```python
from build123d import *

# Parameters (mm, degrees)
SKETCH1_W           = 30
SKETCH1_H           = 99.95
BOSS_EXTRUDE1_DEPTH = 3.75
SKETCH2_W           = 30
SKETCH2_H           = 5
BOSS_EXTRUDE2_DEPTH = 20
SKETCH3_W           = 30
SKETCH3_H           = 5
BOSS_EXTRUDE3_DEPTH = 10
FILLET1_R           = 10
FILLET2_R           = 10


with BuildPart() as part:
    # Sketch1 → Boss-Extrude1 (new, symmetric)
    with BuildSketch(Plane.XY):
        with Locations((0, 49.975)):
            Rectangle(SKETCH1_W, SKETCH1_H)
    extrude(amount=BOSS_EXTRUDE1_DEPTH, both=True)

    # Sketch2 → Boss-Extrude2 (add, symmetric)
    with BuildSketch(Plane.XY):
        with Locations((0, 2.5)):
            Rectangle(SKETCH2_W, SKETCH2_H)
    extrude(amount=BOSS_EXTRUDE2_DEPTH, both=True)

    # Sketch3 → Boss-Extrude3 (add, symmetric)
    with BuildSketch(Plane.XY):
        with Locations((0, 97.45)):
            Rectangle(SKETCH3_W, SKETCH3_H)
    extrude(amount=BOSS_EXTRUDE3_DEPTH, both=True)

    # Fillet1
    # the kernel refuses this fillet: 10 mm, written as the material it adds along each edge
    with BuildSketch(Plane(origin=(15, 94.95, -3.75), x_dir=(0, 0, -1), z_dir=(-1, 0, 0))) as fillet1_piece_1:
        with BuildLine():
            CenterArc((10, 9.270248109), FILLET1_R, 180, 67.975687163)
            Line((0, 9.270248109), (-0.2, 9.270248109))
            Line((-0.2, 9.270248109), (-0.2, 0))
            Line((-0.2, 0), (0, -0.2))
            ThreePointArc((0, -0.2), (3.125, -0.2), (6.175, -0.185404962))
            Line((6.175, -0.185404962), (6.25, 0))
        make_face()
    extrude(amount=30)
    with BuildSketch(Plane(origin=(15, 94.95, 3.75), x_dir=(0, -1, 0), z_dir=(-1, 0, 0))) as fillet1_piece_2:
        with BuildLine():
            CenterArc((9.270248109, 10), FILLET1_R, 202.024312837, 67.975687163)
            Line((0, 6.25), (-0.185404962, 6.175))
            ThreePointArc((-0.185404962, 6.175), (-0.2, 3.125), (-0.2, 0))
            Line((-0.2, 0), (0, -0.2))
            Line((0, -0.2), (9.270248109, -0.2))
            Line((9.270248109, -0.2), (9.270248109, 0))
        make_face()
    extrude(amount=30)

    # Fillet2
    fillet2_edges = [part.edges().sort_by_distance(p)[0] for p in [
        (0, 5, -3.75),
        (0, 5, 3.75),
    ]]
    fillet(fillet2_edges, radius=FILLET2_R)


solid = part.part
```
Geometry check sheet. Reference: the model listing, model coordinates, mm. A direction names the side the tool comes from. Round coordinates to 2 decimals unless told otherwise and drop trailing zeros. Order: outer loops, then holes, each group sorted by start corner. A loop starts at its lowest first (then second) coordinate and runs counter-clockwise, first axis right, second up. Notation, with made-up numbers: (6.5, 84.25) - (53.5, 84.25) arc R22 ccw to (53.5, 106.25) - close; hole circle Ø6 at (84, -16). An arc over 180 degrees is marked (long way). Use a Markdown table: item, result. Add a question column.
1) Gauge pin test, flat ends, axial feed: P1, Ø5, axis at x = 6, z = -15.5, coming from the +Y side; P2, Ø2.5, axis at x = -3, y = 96.5, coming from the +Z side; P3, Ø5, axis at x = -2, y = 51, coming from the +Z side. Record the tip position at first contact, or that the pin passes through.
2) Section check A-A (z = -6). Record the cut outline in (x, y), then the cut area to 3 significant figures.
3) Section check D-D (z = -15). Record the cut outline in (x, y), then the cut area to 3 significant figures.
4) Mould release check, pull along Y, two halves, no side actions. Record for faces 5 (the cylindrical face through (0.21, 91.2, -5.41)), 6 (the flat face through (0, 99.95, 0)), 7 (the cylindrical face through (0.21, 8.01, -6.6)), 8 (the flat face through (15, 46, 2)): released by +Y, released by -Y, zero draft, split by the parting line, or undercut.
5) Thickness scan on line 1 along Y through (x, z) = (-4.5, -7); line 2 along Z through (x, y) = (6.5, 32.5); line 3 along Y through (x, z) = (-12.25, 16). Record the ranges inside material, lowest first.
6) Set-up check for faces 1 (the cylindrical face through (0.21, 91.339, 5.505)), 2 (the flat face through (0, 5, -17)), 3 (the flat face through (0, 97, 10)), 4 (the flat face through (0, 51, -3.75)): record each of +Z, -Z, +X, -X, +Y, -Y from which the full face is reachable in a straight line by a thin tool's end or side.
7) Section check C-C (y = 77). Record the cut outline in (x, z).
8) Section check B-B (x = -1.75). Record the cut outline in (y, z), then the cut area to 3 significant figures.
Established:
| question | item | result |
|---|---|---|
| 1 | P1 | y = 5.03 |
| 1 | P2 | z = 10 |
| 1 | P3 | z = 3.75 |
| 2 | outline | (-15, 0) - (15, 0) - (15, 8.68) - (-15, 8.68) - close; (-15, 92) - (15, 92) - (15, 99.95) - (-15, 99.95) - close |
| 2 | area | 499 mm2 |
| 3 | outline | (-15, 0) - (15, 0) - (15, 5) - (-15, 5) - close |
| 3 | area | 150 mm2 |
| 4 | face 5 | undercut |
| 4 | face 6 | released by +Y |
| 4 | face 7 | undercut |
| 4 | face 8 | zero draft |
| 5 | line 1 | 0 to 7.62, 93.06 to 99.95 |
| 5 | line 2 | -3.75 to 3.75 |
| 5 | line 3 | 0 to 5 |
| 6 | face 1 | +Z, +X, -X |
| 6 | face 2 | -Z, +X, -X, +Y |
| 6 | face 3 | +Z, +X, -X, +Y |
| 6 | face 4 | -Z, +X, -X |
| 7 | outline | (-15, -3.75) - (15, -3.75) - (15, 3.75) - (-15, 3.75) - close |
| 8 | outline | (0, -20) - (5, -20) - (5, -13.75) arc R10 cw to (15, -3.75) - (85.68, -3.75) arc R10 cw to (94.95, -10) - (99.95, -10) - (99.95, 10) - (94.95, 10) arc R10 cw to (85.68, 3.75) - (15, 3.75) arc R10 cw to (5, 13.75) - (5, 20) - (0, 20) - close |
| 8 | area | 1,050 mm2 |
